from build123d import *

# Parameters (mm, degrees)
SKETCH1_W           = 21.78773772
SKETCH1_H           = 33
BOSS_EXTRUDE1_DEPTH = 7
SKETCH2_R           = 5
CUT_EXTRUDE1_DEPTH  = 41.158504889
SKETCH3_W           = 10
SKETCH3_H           = 3.5
BOSS_EXTRUDE2_DEPTH = 4.5
SKETCH4_R           = 1
CUT_EXTRUDE2_DEPTH  = 39.434431373
SKETCH5_R           = 1.65
CUT_EXTRUDE3_DEPTH  = 2
FILLET1_R           = 3


with BuildPart() as part:
    # Sketch1 → Boss-Extrude1 (new body)
    with BuildSketch(Plane.XY):
        with Locations((10.89386886, 16.5)):
            Rectangle(SKETCH1_W, SKETCH1_H)
    extrude(amount=BOSS_EXTRUDE1_DEPTH)

    # Sketch2 → Cut-Extrude1 (cut, through all)
    with BuildSketch(Plane.XY.offset(7)):
        with Locations((10.89386886, 25)):
            Circle(SKETCH2_R)
    extrude(amount=-CUT_EXTRUDE1_DEPTH, mode=Mode.SUBTRACT)

    # Sketch3 → Boss-Extrude2 (add)
    with BuildSketch(Plane.XY.offset(7)):
        with Locations((10.89386886, 1.75)):
            Rectangle(SKETCH3_W, SKETCH3_H)
    boss_extrude2 = extrude(amount=BOSS_EXTRUDE2_DEPTH)

    # Mirror1: Boss-Extrude2 across plane
    add(boss_extrude2.mirror(Plane.XY.offset(3.5)))

    # Sketch4 → Cut-Extrude2 (cut, through all)
    with BuildSketch(Plane(origin=(0, 3.5, 0), x_dir=(1, 0, 0), z_dir=(0, 1, 0))):
        with Locations(Location((10.89386886, 2.25, 0), (0, 0, 180))):
            Circle(SKETCH4_R)
        with Locations(Location((10.89386886, -9.25, 0), (0, 0, 180))):
            Circle(SKETCH4_R)
    extrude(amount=-CUT_EXTRUDE2_DEPTH, mode=Mode.SUBTRACT)

    # Sketch5 → Cut-Extrude3 (cut)
    with BuildSketch(Plane(origin=(0, 3.5, 0), x_dir=(1, 0, 0), z_dir=(0, 1, 0))):
        with Locations(Location((10.89386886, 2.25, 0), (0, 0, 180))):
            Circle(SKETCH5_R)
        with Locations(Location((10.89386886, -9.25, 0), (0, 0, 180))):
            Circle(SKETCH5_R)
    extrude(amount=-CUT_EXTRUDE3_DEPTH, mode=Mode.SUBTRACT)

    # Fillet1
    # the kernel refuses this fillet: 3 mm, written as the material it adds along each edge
    with BuildSketch(Plane(origin=(15.89386886, 3.5, 7), x_dir=(0, 1, 0), z_dir=(-1, 0, 0))) as fillet1_piece_1_section:
        with BuildLine():
            CenterArc((FILLET1_R, -FILLET1_R), FILLET1_R, 90, 90)
            Line((0, -FILLET1_R), (0, 0))
            Line((0, 0), (FILLET1_R, 0))
        make_face()
    fillet1_piece_1 = extrude(amount=10, mode=Mode.PRIVATE)
    fillet1_piece_1 = fillet1_piece_1 - Plane(origin=(10.89386886, 4.228948509, 9.25), x_dir=(-1, 0, 0), z_dir=(0, 1, 0)) * Cylinder(1.65, 32, mode=Mode.PRIVATE)
    add(fillet1_piece_1)
    with BuildSketch(Plane(origin=(15.89386886, 3.5, 0), x_dir=(0, 1, 0), z_dir=(-1, 0, 0))) as fillet1_piece_2_section:
        with BuildLine():
            CenterArc((FILLET1_R, FILLET1_R), FILLET1_R, 180, 90)
            Line((0, FILLET1_R), (0, 0))
            Line((0, 0), (FILLET1_R, 0))
        make_face()
    fillet1_piece_2 = extrude(amount=10, mode=Mode.PRIVATE)
    fillet1_piece_2 = fillet1_piece_2 - Plane(origin=(10.89386886, 4.228948802, -2.25), x_dir=(-1, 0, 0), z_dir=(0, 1, 0)) * Cylinder(1.65, 32, mode=Mode.PRIVATE)
    add(fillet1_piece_2)


solid = part.part
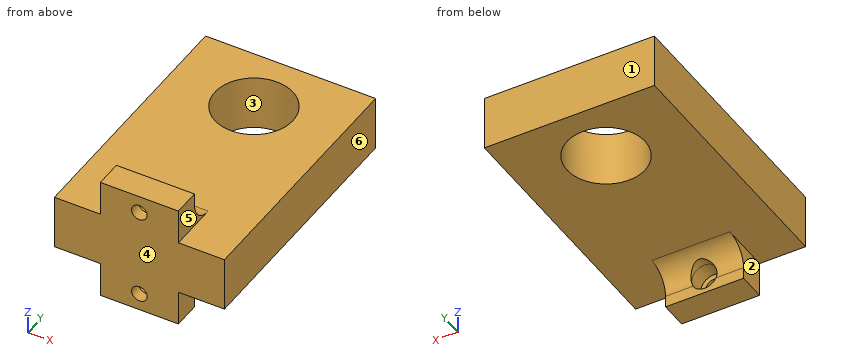
Source: CAD feature listing. Evaluate the final solid. Frame: model axes, mm. Face numbers are marked on the shaded views. A direction names the side the tool comes from. Round coordinates to 2 decimals unless told otherwise and drop trailing zeros. Write each loop counter-clockwise with the first axis right and the second up, starting at its lowest first coordinate (ties: lowest second). Pieces come first, ordered by that corner, then holes. Notation, with made-up numbers: (86, 57.25) - (114, 57.25) arc R21 ccw to (114, 91.25) - close; hole circle Ø11 at (8.5, 1). An arc over 180 degrees is marked (long way). Use CSV: the item, a comma, the result in double quotes. Start each with the question number.
(1) Set-up query: the marked faces 5 and 6. Return all of +Z, -Z, +X, -X, +Y, -Y with unobstructed straight access to the full face (end or side cutting, diameter ignored); none if empty.
(2) Cut plane A-A, the plane y = 25. Return loops of the section in (x, z).
(3) Material intervals for probe 1 along Z at (x, y) = (13, 19.5); probe 2 along Y at (x, z) = (7, 3); probe 3 along Y at (x, z) = (10.5, 2.75), sorted ascending. Write a range as [from, to].
(4) First-contact query: pin 1 Ø2.5 at (x, z) = (11.5, -2.5) entering from +Y; pin 2 Ø1 at (x, y) = (4.5, 21.5) entering from +Z; pin 3 Ø5 at (y, z) = (2, 10) entering from -X. Flat tips, straight axial feed; report the tip coordinate or a pass-through.
(5) Cut plane B-B, the plane z = 2. Return loops of the section in (x, y), and give its area (3 significant figures).
(6) Mould query, pull axis Y, two halves, no side actions, for the marked faces 1, 2, 3 and 4. Classes: pulls with the +Y half, pulls with the -Y half, needs draft (parallel to the pull), parting line crosses it, or undercut.
(7) Cut plane C-C, the plane z = 9.25. Return loops of the section in (x, y), and give its area (3 significant figures).
(8) Cut plane D-D, the plane x = 17. Return loops of the section in (y, z).
Geometry says:
1,face 5,"+Z, +X, +Y, -Y"
1,face 6,"+Z, -Z, +X, +Y, -Y"
2,outline,"(0, 0) - (5.89, 0) - (5.89, 7) - (0, 7) - close; (15.89, 0) - (21.79, 0) - (21.79, 7) - (15.89, 7) - close"
3,probe 1,"[0, 7]"
3,probe 2,"[0, 21.86], [28.14, 33]"
3,probe 3,"[0, 20.02], [29.98, 33]"
4,pin 1,"y = 3.81"
4,pin 2,"z = 7"
4,pin 3,"x = 5.89"
5,outline,"(0, 0) - (21.79, 0) - (21.79, 33) - (0, 33) - close; hole circle Ø10 at (10.89, 25)"
5,area,"640 mm²"
6,face 1,"pulls with the +Y half"
6,face 2,"needs draft"
6,face 3,"undercut"
6,face 4,"pulls with the -Y half"
7,outline,"(5.89, 0) - (9.89, 0) - (9.89, 1.5) - (9.24, 1.5) - (9.24, 3.6) - (5.89, 3.6) - close; (11.89, 0) - (15.89, 0) - (15.89, 3.6) - (12.54, 3.6) - (12.54, 1.5) - (11.89, 1.5) - close"
7,area,"26.0 mm²"
8,outline,"(0, 0) - (33, 0) - (33, 7) - (0, 7) - close"
